Work out the finished part from the listing and answer in its coordinate system (mm). A direction names the side the tool comes from. Round coordinates to 2 decimals unless told otherwise and drop trailing zeros. Order: outer loops, then holes, each group sorted by start corner. A loop starts at its lowest first (then second) coordinate and runs counter-clockwise, first axis right, second up. Notation, with made-up numbers: M -10.5,72.5 L 4.5,72.5 A26 ccw 4.5,97.5 Z; hole C 62.25,19 d10. An arc over 180 degrees is marked long. Return JSON: item names as keys, results as strings.
from build123d import *

# Parameters (mm, degrees)
SKETCH1_R           = 275
BOSS_EXTRUDE1_DEPTH = 160
FILLET1_R           = 50
SKETCH2_R           = 25
CUT_EXTRUDE1_DEPTH  = 50
SKETCH3_R           = 125
CUT_EXTRUDE2_DEPTH  = 20
SKETCH4_W           = 26.72203761
SKETCH4_H           = 21.282518002
BOSS_EXTRUDE2_DEPTH = 77


with BuildPart() as part:
    # Sketch1 → Boss-Extrude1 (new body)
    with BuildSketch(Plane(origin=(0, 0, 0), x_dir=(0, 0, -1), z_dir=(1, 0, 0))):
        Circle(SKETCH1_R)
    extrude(amount=BOSS_EXTRUDE1_DEPTH)

    # Fillet1
    fillet1_edges = [part.edges().sort_by_distance(p)[0] for p in [
        (0, 0, 275),
        (160, 0, 275),
    ]]
    fillet(fillet1_edges, radius=FILLET1_R)

    # Sketch2 → Cut-Extrude1 (cut)
    with BuildSketch(Plane.ZY):
        Circle(SKETCH2_R)
    extrude(amount=-CUT_EXTRUDE1_DEPTH, mode=Mode.SUBTRACT)

    # Sketch3 → Cut-Extrude2 (cut)
    with BuildSketch(Plane(origin=(160, 0, 0), x_dir=(0, 0, -1), z_dir=(1, 0, 0))):
        Circle(SKETCH3_R)
    extrude(amount=-CUT_EXTRUDE2_DEPTH, mode=Mode.SUBTRACT)

    # Sketch4 → Boss-Extrude2 (add)
    with BuildSketch(Plane(origin=(160, 0, 0), x_dir=(0, 0, -1), z_dir=(1, 0, 0))):
        with Locations((0, -125)):
            Rectangle(SKETCH4_W, SKETCH4_H)
        Polygon((-56.409090154, -100.371574733), (-68.918640367, -117.58949348), (-90.537222919, -101.882673861), (-78.027672706, -84.664755114), align=None)
        Polygon((-104.632843949, -48.045878423), (-124.873721378, -54.622538169), (-133.131285124, -29.208370171), (-112.890407695, -22.631710425), align=None)
        Polygon((-112.890407695, 22.631710425), (-133.131285124, 29.208370171), (-124.873721378, 54.622538169), (-104.632843949, 48.045878423), align=None)
        Polygon((-78.027672706, 84.664755114), (-90.537222919, 101.882673861), (-68.918640367, 117.58949348), (-56.409090154, 100.371574733), align=None)
        with Locations((0, 125)):
            Rectangle(SKETCH4_W, SKETCH4_H)
        Polygon((56.409090154, 100.371574733), (68.918640368, 117.58949348), (90.537222919, 101.882673861), (78.027672706, 84.664755114), align=None)
        Polygon((104.632843949, 48.045878423), (124.873721378, 54.622538169), (133.131285124, 29.208370171), (112.890407695, 22.631710425), align=None)
        Polygon((112.890407695, -22.631710425), (133.131285124, -29.208370171), (124.873721378, -54.622538169), (104.632843949, -48.045878423), align=None)
        Polygon((78.027672706, -84.664755114), (90.537222919, -101.882673861), (68.918640367, -117.58949348), (56.409090154, -100.371574733), align=None)
    extrude(amount=-BOSS_EXTRUDE2_DEPTH)


solid = part.part
Item 1: Find section A-A (y = 0). Determine the outline of the cut face in (x, z), plus the area to 3 significant figures.
Output:
{"outline": "M 0,-225 A50 ccw 50,-275 L 110,-275 A50 ccw 160,-225 L 160,-125 L 140,-125 L 140,125 L 160,125 L 160,225 A50 ccw 110,275 L 50,275 A50 ccw 0,225 L 0,25 L 50,25 L 50,-25 L 0,-25 Z", "area": "78,400 mm^2"}
Item 2: Consider line 1 along Y through (x, z) = (30, 0); line 2 along Y through (x, z) = (22.5, 0); line 3 along X through (y, z) = (224.5, 118.5). Determine where each line is inside the solid, lowest interval first. Write a range as [from, to].
Output:
{"line 1": "y = [-270.83, -25], [25, 270.83]", "line 2": "y = [-266.76, -25], [25, 266.76]", "line 3": "x = [9.17, 150.83]"}
Item 3: Find section D-D (x = 36.5). Determine the outline of the cut face in (y, z), plus the area to 3 significant figures.
Output:
{"outline": "C 0,0 d546.29; hole C 0,0 d50", "area": "232,000 mm^2"}
Item 4: The mould has two halves that part along Z. Classify faces 3 (the cylindrical face through (150.14, -73.18, 101.34)), 4 (the flat face through (160, -97, -97)): pulls with the +Z half, pulls with the -Z half, needs draft (parallel to the pull), parting line crosses it, or undercut.
Output:
{"face 3": "undercut", "face 4": "needs draft"}
Item 5: Find section C-C (x = 74.5). Determine the outline of the cut face in (y, z).
Output:
{"outline": "C 0,0 d550"}
Item 6: Find section B-B (z = 0). Determine the outline of the cut face in (x, y).
Output:
{"outline": "M 0,-225 A50 ccw 50,-275 L 110,-275 A50 ccw 160,-225 L 160,-114.36 L 140,-114.36 L 140,114.36 L 160,114.36 L 160,225 A50 ccw 110,275 L 50,275 A50 ccw 0,225 L 0,25 L 50,25 L 50,-25 L 0,-25 Z"}
Item 7: Each of these flat-tipped pins is pushed along its axis until it touches: pin 1 (1 mm diameter, centred on y = -219, z = -150.5, fed in from -X); pin 2 (11 mm diameter, centred on x = 149.5, y = 117, fed in from -Z); pin 3 (6 mm diameter, centred on x = 110.5, z = 69, fed in from +Y). Where does it stop, or does it pass through?
Output:
{"pin 1": "stops at x = 20.31", "pin 2": "stops at z = -234.65", "pin 3": "stops at y = 266.96"}
Item 8: Which of the six approach directions +Z, -Z, +X, -X, +Y, -Y give full straight-line access (tool end or side, diameter ignored) to faces 1 (the flat face through (0, -47, 3)), 2 (the flat face through (150.14, 92.41, -67.37))?
Output:
{"face 1": "+Z, -Z, -X, +Y, -Y", "face 2": "+X"}
